Build history of the part. All positions in model axes, mm. A direction names the side the tool comes from. Round coordinates to 2 decimals unless told otherwise and drop trailing zeros. Write each loop counter-clockwise with the first axis right and the second up, starting at its lowest first coordinate (ties: lowest second). Pieces come first, ordered by that corner, then holes.
1) Saw through at D-D (z = 0.5). Write the cut outline in (x, y).
2) Which spindle directions (+Z, -Z, +X, -X, +Y, -Y) get a long thin tool onto all of the face, cutting with end or side? Do faces 1 (the flat face through (5, -3, 0.3)), 2 (the cylindrical face through (-4.806, -4.765, 1.396)), 3 (the cylindrical face through (14.2, -3.5, 0.5)). Say none if no direction does.
3) Pull direction X, two halves, no side cores. Call faces 4 (the flat face through (-5.5, -3.5, 0.8)), 5 (the flat face through (12.85, -2.92, 0)), 6 (the flat face through (-5, -4, 1)): +X half, -X half, draft (parallel to the pull), parting line (faces both ways), or undercut.
4) Flat gauge pins, fed straight in: pin 1 (1 mm diameter, centred on x = 0.5, z = 0.5, fed in from -Y); pin 2 (1.5 mm diameter, centred on x = -3.5, y = -4, fed in from +Z). Where does each tip first touch, or does it go through?
5) Saw through at B-B (y = -3.9). Write the cut outline in (x, z).
6) Wall check: probe 1 along X at (y, z) = (-4.3, 1.35); probe 2 along X at (y, z) = (-4.6, 1.5); probe 3 along Y at (x, z) = (2, 1.5). Give the ranges that are in metal, low to high.
7) Saw through at C-C (x = -4). Write the cut outline in (y, z).
Autodesk Inventor part; units mm, degrees
ref_plane "作業平面2" through (-5.5, -5.9495, 0) normal (1, 0, 0) x (0, 1, 0)
ref_plane "作業平面3" through (12, 0, -1) normal (0, 0, -1) x (-1, 0, 0)
ref_plane "作業平面5" through (15, -3.5, 1) normal (0, 0, -1) x (-1, 0, 0)
ref_plane "作業平面1" through (15, -6, 0) normal (-1, 0, 0) x (0, -1, 0)
sketch "スケッチ1" plane through (15, -6, 0) normal (-1, 0, 0) x (0, -1, 0)
  arc A0 (-0.0505, 0) -> (-4.9495, 0) centre (-2.5, -0.5) ccw
  line L0 (-4.9495, 0) -> (-0.0505, 0)
  point P0 (-6, 0)
ref_plane "作業平面2" through (-5.5, -5.9495, 0) normal (1, 0, 0) x (0, 1, 0)
extrude "押し出し1" add sketch "スケッチ1" along normal up to surface (20.5 mm away)
ref_plane "作業平面3" through (12, 0, -1) normal (0, 0, -1) x (-1, 0, 0)
sketch "スケッチ2" plane through (12, 0, 0) normal (0, 0, -1) x (-1, 0, 0)
  line L0 (14.5, -5.9495) -> (17.5, -5.9495) construction
  line L1 (14.5, -1.0505) -> (14.5, -5.9495) construction
  line L2 (17.5, -1.0505) -> (14.5, -1.0505) construction
  line L3 (17.5, -5.9495) -> (17.5, -1.0505) construction
  arc A0 (0, -3) -> (0.5, -3.5) centre (0.5, -3) ccw construction
  line L4 (0.5, -3.5) -> (7.401, -3.5) construction
  arc A1 (7.401, -3.5) -> (7.901, -3) centre (7.401, -3) ccw construction
  line L5 (7.901, -3) -> (7.901, -2.5) construction
  arc A2 (7.901, -2.5) -> (7.401, -2) centre (7.401, -2.5) ccw construction
  line L6 (7.401, -2) -> (0.5, -2) construction
  arc A3 (0.5, -2) -> (0, -2.5) centre (0.5, -2.5) ccw construction
  line L7 (0, -3) -> (0, -2.5) construction
  spline S0 degree 3 poles (8.201, -0.8167) (8.2004, -0.8173) (8.1998, -0.8179) (8.1567, -0.8609) (8.1131, -0.8989) (8.0137, -0.9678) (7.9594, -0.997) (7.8435, -1.0385) (7.7825, -1.0505) (7.721, -1.0505) knots -0.000247 -0.000247 -0.000247 -0.000247 0 0 0.018039 0.018039 0.036793 0.036793 0.055658 0.055658 0.055658 0.055658 construction
  line L8 (8.201, -0.3) -> (8.201, -0.8167) construction
  line L9 (11.7, -0.3) -> (8.201, -0.3) construction
  line L10 (11.7, -4.5) -> (11.7, -0.3) construction
  line L11 (11.7, -4.5) -> (0.3, -4.5) construction
  arc A4 (0.3, -4.5) -> (0, -4.8) centre (0.3, -4.8) ccw construction
  line L12 (0, -5.9495) -> (0, -4.8) construction
  line L13 (-3, -5.9495) -> (0, -5.9495) construction
  line L14 (-3, -1.0505) -> (-3, -5.9495) construction
  line L15 (7.721, -1.0505) -> (-3, -1.0505) construction
  line L16 (17.5, -1.0505) -> (17.5, -5.9495) construction
  line L17 (-3, -1.0505) -> (17.5, -1.0505) construction
  line L18 (-3, -5.9495) -> (-3, -1.0505) construction
  line L19 (-3, -5.9495) -> (17.5, -5.9495) construction
  line L20 (14.5, -5.9495) -> (0, -5.9495)
  line L21 (0, -5.9495) -> (0, -1.0505)
  line L22 (0, -1.0505) -> (14.5, -1.0505)
  line L23 (14.5, -1.0505) -> (14.5, -5.9495)
  circle A5 centre (16, -3.5) radius 0.55
  circle A6 centre (-1.5, -3.5) radius 0.55
  point P0 (12, 0)
extrude "押し出し2" cut sketch "スケッチ2" against normal blind 0.3 contours L20 L21 L22 L23
sketch "スケッチ3" plane through (15, -5.9495, 0) normal (0, 0, -1) x (-1, 0, 0)
  line L0 (17.5, 4.899) -> (17.5, 0) construction
  line L1 (17.5, 0) -> (20.5, 0) construction
  line L2 (20.5, 4.899) -> (20.5, 0) construction
  line L3 (17.5, 4.899) -> (20.5, 4.899) construction
  line L4 (3, 0) -> (3, 4.899) construction
  line L5 (0, 4.899) -> (3, 4.899) construction
  line L6 (0, 0) -> (0, 4.899) construction
  line L7 (0, 0) -> (3, 0) construction
  line L8 (20.5, 0) -> (20.5, 4.899) construction
  line L9 (20.5, 0) -> (17.5, 4.899) construction
  line L10 (17.5, 0) -> (20.5, 0) construction
  line L11 (17.5, 0) -> (20.5, 4.899) construction
  line L12 (0, 0) -> (0, 4.899) construction
  line L13 (3, 4.899) -> (0, 0) construction
  line L14 (0, 4.899) -> (3, 4.899) construction
  line L15 (0, 0) -> (0, 4.899) construction
  line L16 (3, 0) -> (3, 4.899) construction
  line L17 (0, 4.899) -> (3, 0) construction
  circle A0 centre (19, 2.4495) radius 0.7
  circle A1 centre (1.5, 2.4495) radius 0.7
  point P0 (15, 5.9495)
  dimension "d5" = 1.4
extrude "押し出し3" cut sketch "スケッチ3" against normal up to next
ref_plane "作業平面5" through (15, -3.5, 1) normal (0, 0, -1) x (-1, 0, 0)
ref_plane "作業平面4" through (15, -3.5, 2) normal (0, 0, -1) x (-1, 0, 0)
sketch "スケッチ4" plane through (15, -3.5, 2) normal (0, 0, -1) x (-1, 0, 0)
  circle A0 centre (19, 0) radius 1.5
  circle A1 centre (1.5, 0) radius 0.7
  circle A2 centre (1.5, 0) radius 1.5
  circle A3 centre (19, 0) radius 0.7
  point P0 (15, 3.5)
  point P1 (19, 0.7)
  point P2 (1.5, 0.7)
  dimension "d9" = 3
extrude "押し出し4" cut sketch "スケッチ4" along normal up to surface (1 mm away) contours A0 | A1 | A2 | A3
properties part number "SR-T-09"
Evaluation:
1. outline: (-5.5, -5.79) - (15, -5.79) - (15, -1.21) - (-5.5, -1.21) - close; hole circle Ø1.4 at (-4, -3.5); hole circle Ø1.4 at (13.5, -3.5)
2. face 1: -Z, +Y, -Y
2. face 2: +Z
2. face 3: +Z, -Z
3. face 4: -X half
3. face 5: draft
3. face 6: undercut
4. pin 1: stops at y = -5.87
4. pin 2: stops at z = 1
5. outline: (-5.5, 0) - (-4.57, 0) - (-4.57, 1) - (-5.45, 1) - (-5.45, 1.97) - (-5.5, 1.97) - close; (-3.43, 0) - (-2.5, 0) - (-2.5, 0.3) - (12, 0.3) - (12, 0) - (12.93, 0) - (12.93, 1) - (12.05, 1) - (12.05, 1.97) - (-2.55, 1.97) - (-2.55, 1) - (-3.43, 1) - close; (14.07, 0) - (15, 0) - (15, 1.97) - (14.95, 1.97) - (14.95, 1) - (14.07, 1) - close
6. probe 1: x = -5.5 to -5.27, -2.73 to 12.23, 14.77 to 15
6. probe 2: x = -5.5 to -5.02, -2.98 to 12.48, 14.52 to 15
6. probe 3: y = -5 to -2
7. outline: (-5.95, 0) - (-4.2, 0) - (-4.2, 1) - (-5, 1) - (-5, 1.5) arc R2.5 ccw to start; (-2.8, 0) - (-1.05, 0) arc R2.5 ccw to (-2, 1.5) - (-2, 1) - (-2.8, 1) - close
